Source: CAD feature listing. Evaluate the final solid. Frame: model axes, mm. Face numbers are marked on the shaded views. A direction names the side the tool comes from. Round coordinates to 2 decimals unless told otherwise and drop trailing zeros. Order: outer loops, then holes, each group sorted by start corner. A loop starts at its lowest first (then second) coordinate and runs counter-clockwise, first axis right, second up. Notation, with made-up numbers: M -25,85.25 L -3,85.25 A23 cw -3,109.25 Z; hole C 35,53 d1. An arc over 180 degrees is marked long. Use one line per item in the form item = value. Start each with the question number.
Q1. Contact query for flat-ended pins moving along their axis: pin 1 (10 mm diameter, centred on y = -5.5, z = 14, fed in from -X); pin 2 (4 mm diameter, centred on y = -8, z = 14, fed in from -X); pin 3 (6 mm diameter, centred on y = -14, z = 13, fed in from -X). Output: stop coordinate, or through.
Q2. Material intervals for probe 1 along Z at (x, y) = (2.75, -13); probe 2 along Y at (x, z) = (0, 3.75); probe 3 along X at (y, z) = (-17.75, 3), sorted ascending.
Q3. Pull-direction query (Y, two-part tool) for the marked faces 4, 5, 6 and 7; classes: pulls with the +Y half, pulls with the -Y half, needs draft (parallel to the pull), parting line crosses it, or undercut.
Q4. Section B-B (y = -8.25). Return the cut outline in (x, z).
Q5. Section A-A (x = -5.5). Return the cut outline in (y, z), plus the area to 3 significant figures.
Q6. Section D-D (z = 8). Return the cut outline in (x, y).
Q7. Reachability of the marked faces 1, 2 and 3 from +Z, -Z, +X, -X, +Y, -Y: full face, straight path, thin tool, end or side. Return the list, or none.
Q8. Section C-C (x = 0). Return the cut outline in (y, z).
from build123d import *

# Parameters (mm, degrees)
F0_R     = 1.5
F1_DEPTH = 18
F2_W     = 16.085666
F2_H     = 3
F3_DEPTH = 11


with BuildPart() as f1:
    # F0 (on Top) → F1 (new body)
    with BuildSketch(Plane.XY):
        with BuildLine():
            Line((4.330127, -1.25), (5, -1.25))
            Line((5, -1.25), (5, 1.25))
            Line((5, 1.25), (-5, 1.25))
            Line((-5, 1.25), (-5, -1.25))
            Line((-5, -1.25), (-4.330127, -1.25))
            ThreePointArc((-4.330127, -1.25), (-4.953899, -4.42741), (-3.5, -7.320714))
            Line((-3.5, -7.320714), (-3.5, -18.75))
            Line((-3.5, -18.75), (-6, -18.75))
            Line((-6, -18.75), (-6, -20.75058))
            Line((-6, -20.75058), (5, -20.75058))
            Line((5, -20.75058), (5, -18.75))
            Line((5, -18.75), (5, -3.75))
            ThreePointArc((5, -3.75), (4.829629, -2.455905), (4.330127, -1.25))
        make_face()
        with Locations((0, -17.75058)):
            Circle(F0_R, mode=Mode.SUBTRACT)
    extrude(amount=F1_DEPTH)

    # F2 (on face) → F3 (cut)
    with BuildSketch(Plane.YZ.offset(5)):
        with Locations((-12.707747, 9)):
            Rectangle(F2_W, F2_H)
    extrude(amount=-F3_DEPTH, mode=Mode.SUBTRACT)


solid = f1.part
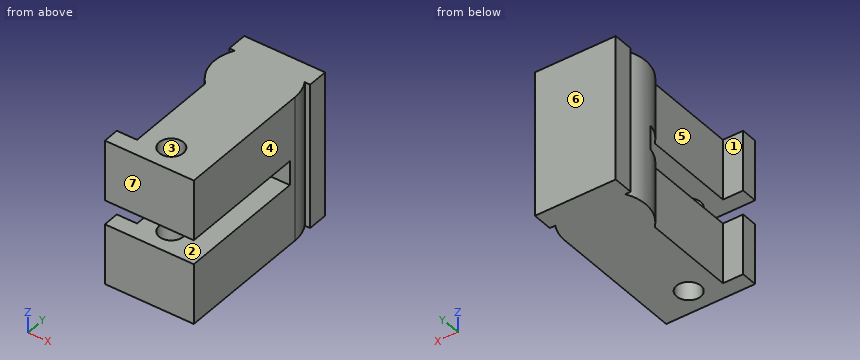
Results list:
q1.pin_1 = -5
q1.pin_2 = -4.47
q1.pin_3 = -3.5
q2.probe_1 = 0 to 7.5, 10.5 to 18
q2.probe_2 = -20.75 to -19.25, -16.25 to 1.25
q2.probe_3 = -3.5 to -1.5, 1.5 to 5
q3.face_4 = needs draft
q3.face_5 = undercut
q3.face_6 = pulls with the +Y half
q3.face_7 = pulls with the -Y half
q4.outline = M -3.5,0 L 5,0 L 5,7.5 L -3.5,7.5 Z; M -3.5,10.5 L 5,10.5 L 5,18 L -3.5,18 Z
q5.outline = M -20.75,0 L -18.75,0 L -18.75,7.5 L -20.75,7.5 Z; M -20.75,10.5 L -18.75,10.5 L -18.75,18 L -20.75,18 Z
q5.area = 30.0 mm2
q6.outline = M -5,-1.25 L -4.33,-1.25 A5 ccw -4.92,-4.66 L 5,-4.66 L 5,-3.75 A5 ccw 4.33,-1.25 L 5,-1.25 L 5,1.25 L -5,1.25 Z
q7.face_1 = +Z, -Z, -X
q7.face_2 = +X, -X, -Y
q7.face_3 = +Z, -Z
q8.outline = M -20.75,0 L -19.25,0 L -19.25,7.5 L -20.75,7.5 Z; M -20.75,10.5 L -19.25,10.5 L -19.25,18 L -20.75,18 Z; M -16.25,0 L 1.25,0 L 1.25,18 L -16.25,18 L -16.25,10.5 L -4.66,10.5 L -4.66,7.5 L -16.25,7.5 Z
